Part model, mm, in its own coordinate system. Face numbers are marked on the shaded views. A direction names the side the tool comes from. Give positions to 0.01 mm unless a question says otherwise; leave off trailing zeros. Write each loop counter-clockwise with the first axis right and the second up, starting at its lowest first coordinate (ties: lowest second). Pieces come first, ordered by that corner, then holes. Notation, with made-up numbers: M 46,22.25 L 102,22.25 A8 cw 102,31.25 Z; hole C 6.25,14 d4. An arc over 180 degrees is marked long. Write item = value, one per line. Start each with the question number.
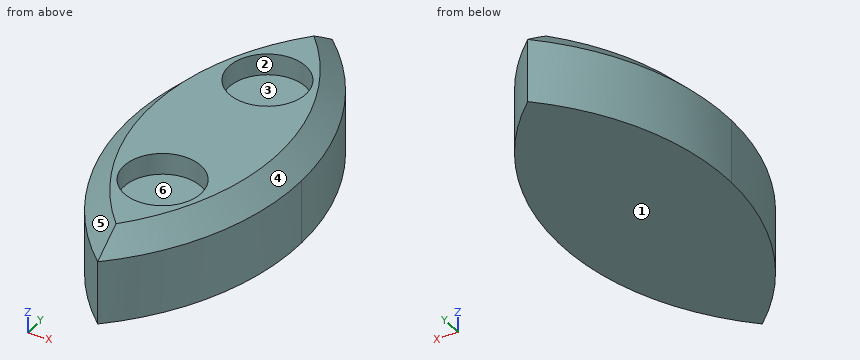
from build123d import *

# Parameters (mm, degrees)
F0_R        = 9
F1_DEPTH    = 20
F2_DEPTH    = 15
F3_T2_ANGLE = 120.9484473771
F3_T4_ANGLE = 120.9484473771


# Not quite as in the source:
# - a fillet or chamfer that OpenCascade refuses, or shapes differently, is made with other operations: its cross-section is extruded or revolved along the edge and cut away or added


with BuildPart() as f1:
    # F0 (on Top) → F1 (new body)
    with BuildSketch(Plane.XY):
        with BuildLine():
            Line((-20, 0), (0, 0))
            Line((0, 0), (20, 0))
            ThreePointArc((20, 0), (14.7722557505, 24.4948974278), (0, 44.72135955))
            ThreePointArc((0, 44.72135955), (-14.7722557505, 24.4948974278), (-20, 0))
        make_face()
        with Locations((0, 20)):
            Circle(F0_R, mode=Mode.SUBTRACT)
        with BuildLine():
            Line((20, 0), (0, 0))
            Line((0, 0), (-20, 0))
            ThreePointArc((-20, 0), (-14.7722557505, -24.4948974278), (0, -44.72135955))
            ThreePointArc((0, -44.72135955), (14.7722557505, -24.4948974278), (20, 0))
        make_face()
        with Locations((0, -20)):
            Circle(F0_R, mode=Mode.SUBTRACT)
    extrude(amount=F1_DEPTH)

    # F0 (on Top) → F2 (join)
    with BuildSketch(Plane.XY):
        with Locations((0, -20)):
            Circle(F0_R)
        with Locations((0, 20)):
            Circle(F0_R)
    extrude(amount=F2_DEPTH)

    # F3: chamfer of 5 on 2 edges, made by hand

    # F3_s1 → F3_t2 (revolve, cut)
    with BuildSketch(Plane(origin=(-30.2853323821, -17.1526073175, 0), x_dir=(0, 0, 1), z_dir=(-0.8701340756, -0.4928150672, 0))):
        Polygon((15, -40.2873973125), (20, -35.2873973125), (20, -40.2873973125), align=None)
    revolve(axis=Axis((-40, 0, 20), (0, 0, 1)), revolution_arc=F3_T2_ANGLE, mode=Mode.SUBTRACT)

    # F3_s3 → F3_t4 (revolve, cut)
    with BuildSketch(Plane(origin=(30.2853323821, 17.1526073175, 0), x_dir=(0, 0, 1), z_dir=(0.8701340756, 0.4928150672, 0))):
        Polygon((15, -40.2873973125), (20, -35.2873973125), (20, -40.2873973125), align=None)
    revolve(axis=Axis((40, 0, 20), (0, 0, 1)), revolution_arc=F3_T4_ANGLE, mode=Mode.SUBTRACT)


solid = f1.part
Q1. Slice it at A-A (z = 1.5). Give the cut face in (x, y), and give its area (3 significant figures).
Q2. Tool access for the marked faces 5 and 6: list every direction of +Z, -Z, +X, -X, +Y, -Y with a clear straight run to the whole face (end or side of a thin tool).
Q3. Drop flat-ended pins along their axis: P1, Ø1.5, axis at y = 23.5, z = 6.5, coming from the +X side; P2, Ø12, axis at x = -7, z = 13.5, coming from the -Y side; P3, Ø1, axis at x = 6.5, y = 17, coming from the +Z side. Give the stop position or say it passes through.
Q4. Slice it at B-B (z = 16.75). Give the cut face in (x, y), and give its area (3 significant figures).
Q5. Two-plate mould, pull along Y, no slides. Class the marked faces 1, 2, 3 and 4: +Y half, -Y half, draft (parallel to the pull), parting line (faces both ways), or undercut.
Q6. Probe line 1 along Y through (x, z) = (0, 18.1); line 2 along Y through (x, z) = (-4, 18.25); line 3 along Z through (x, y) = (-4, -21). List the from-to ranges inside material, lowest first.
Working result:
q1.outline = M 0,-44.72 A60 ccw 0,44.72 A60 ccw Z
q1.area = 2,480 mm2
q2.face_5 = +Z, -X
q2.face_6 = +Z
q3.P1 = 15.52
q3.P2 = -43.81
q3.P3 = 15
q4.outline = M 0,-42.34 A58.25 ccw 0,42.34 A58.25 ccw Z; hole C 0,-20 d18; hole C 0,20 d18
q4.area = 1,630 mm2
q5.face_1 = draft
q5.face_2 = undercut
q5.face_3 = undercut
q5.face_4 = parting line
q6.line_1 = -40.47 to -29, -11 to 11, 29 to 40.47
q6.line_2 = -35.84 to -28.06, -11.94 to 11.94, 28.06 to 35.84
q6.line_3 = 0 to 15
